```python
from build123d import *

# Parameters (mm, degrees)
SKETCH1_W          = 277
SKETCH1_H          = 97.5
BASE_FLANGE1_DEPTH = 1
JOG1_START         = -138.5
JOG1_DEPTH         = 277
JOG1_2_DEPTH       = 277
JOG2_START         = -138.5
JOG2_DEPTH         = 277
JOG2_2_DEPTH       = 277
SKETCH11_W         = 67
SKETCH11_H         = 15
SKETCH11_W_2       = 75
SKETCH11_W_3       = 77
CUT_EXTRUDE1_DEPTH = 148.204152455
SKETCH16_W         = 12
SKETCH16_H         = 22.35
TAB1_DEPTH         = 1
JOG4_START         = 126.5
JOG4_DEPTH         = 12
JOG4_2_DEPTH       = 12
SKETCH22_R         = 1.5
SCREW_HOLES_DEPTH  = 148.204152455
FILLET1_R          = 6
FILLET2_R          = 2


# Read off the part's stored shape, not the designer's step: Jog1, Jog2, Jog4
# Sheet-metal steps are written as plain solids
with BuildPart() as part:
    # Sketch1 → Base-Flange1 (new body)
    with BuildSketch(Plane.XY):
        Rectangle(SKETCH1_W, SKETCH1_H)
    extrude(amount=-BASE_FLANGE1_DEPTH)

    # Jog1 outline → Jog1 (cut)
    with BuildSketch(Plane.YZ.offset(JOG1_START)):
        with BuildLine():
            ThreePointArc((36.928097245, -1), (35.928097245, -0.732050807), (35.196046438, 0))
            Line((35.196046438, 0), (-48.75, 0))
            Line((-48.75, 0), (-48.75, -1))
            Line((-48.75, -1), (36.928097245, -1))
        make_face()
    extrude(amount=JOG1_DEPTH, mode=Mode.SUBTRACT)

    # Jog1 2 outline → Jog1 2 (add)
    with BuildSketch(Plane.YZ.offset(JOG1_START)):
        with BuildLine():
            Line((34.928097245, 7.5), (34.928097245, 1))
            ThreePointArc((34.928097245, 1), (34.996245593, 0.48236191), (35.196046438, 0))
            Line((35.196046438, 0), (36.928097245, 0))
            ThreePointArc((36.928097245, 0), (36.220990464, 0.292893219), (35.928097245, 1))
            Line((35.928097245, 1), (35.928097245, 7.5))
            ThreePointArc((35.928097245, 7.5), (35.342310807, 8.914213562), (33.928097245, 9.5))
            Line((33.928097245, 9.5), (-48.75, 9.5))
            Line((-48.75, 9.5), (-48.75, 8.5))
            Line((-48.75, 8.5), (33.928097245, 8.5))
            ThreePointArc((33.928097245, 8.5), (34.635204026, 8.207106781), (34.928097245, 7.5))
        make_face()
    extrude(amount=JOG1_2_DEPTH)

    # Jog2 outline → Jog2 (cut)
    with BuildSketch(Plane.YZ.offset(JOG2_START)):
        with BuildLine():
            Line((-48.75, 8.5), (-36.303953562, 8.5))
            ThreePointArc((-36.303953562, 8.5), (-35.571902755, 9.232050807), (-34.571902755, 9.5))
            Line((-34.571902755, 9.5), (-48.75, 9.5))
            Line((-48.75, 9.5), (-48.75, 8.5))
        make_face()
    extrude(amount=JOG2_DEPTH, mode=Mode.SUBTRACT)

    # Jog2 2 outline → Jog2 2 (add)
    with BuildSketch(Plane.YZ.offset(JOG2_START)):
        with BuildLine():
            Line((-48.75, -1), (-37.571902755, -1))
            ThreePointArc((-37.571902755, -1), (-36.157689193, -0.414213562), (-35.571902755, 1))
            Line((-35.571902755, 1), (-35.571902755, 7.5))
            ThreePointArc((-35.571902755, 7.5), (-35.279009536, 8.207106781), (-34.571902755, 8.5))
            Line((-34.571902755, 8.5), (-36.303953562, 8.5))
            ThreePointArc((-36.303953562, 8.5), (-36.503754407, 8.01763809), (-36.571902755, 7.5))
            Line((-36.571902755, 7.5), (-36.571902755, 1))
            ThreePointArc((-36.571902755, 1), (-36.864795974, 0.292893219), (-37.571902755, 0))
            Line((-37.571902755, 0), (-48.75, 0))
            Line((-48.75, 0), (-48.75, -1))
        make_face()
    extrude(amount=JOG2_2_DEPTH)

    # Sketch11 → Cut-Extrude1 (cut, through all)
    with BuildSketch(Plane(origin=(0, 0, -1), x_dir=(-1, 0, 0), z_dir=(0, 0, -1))):
        Polygon((-138.5, -48.75), (-123.5, -48.75), (-111.5, -48.75), (47.5, -48.75), (47.5, -33.75), (-111.5, -33.75), (-123.5, -33.75), (-123.5, -28.75), (-138.5, -28.75), align=None)
        with Locations((93, -41.25)):
            Rectangle(SKETCH11_W, SKETCH11_H)
        with Locations((-89, 41.25)):
            Rectangle(SKETCH11_W_2, SKETCH11_H)
        with Locations((-1, 41.25)):
            Rectangle(SKETCH11_W_3, SKETCH11_H)
        with Locations((88, 41.25)):
            Rectangle(SKETCH11_W_3, SKETCH11_H)
    extrude(amount=-CUT_EXTRUDE1_DEPTH, mode=Mode.SUBTRACT)

    # Sketch16 → Tab1 (add)
    with BuildSketch(Plane(origin=(0, 0, 8.5), x_dir=(-1, 0, 0), z_dir=(0, 0, -1))):
        with Locations((-132.5, -39.925)):
            Rectangle(SKETCH16_W, SKETCH16_H)
    extrude(amount=-TAB1_DEPTH)

    # Jog4 outline → Jog4 (cut)
    with BuildSketch(Plane.YZ.offset(JOG4_START)):
        with BuildLine():
            Line((-51.1, 8.5), (-30.986067978, 8.5))
            ThreePointArc((-30.986067978, 8.5), (-29.974744872, 9.238612788), (-28.75, 9.5))
            Line((-28.75, 9.5), (-51.1, 9.5))
            Line((-51.1, 9.5), (-51.1, 8.5))
        make_face()
    extrude(amount=JOG4_DEPTH, mode=Mode.SUBTRACT)

    # Jog4 2 outline → Jog4 2 (add)
    with BuildSketch(Plane.YZ.offset(JOG4_START)):
        with BuildLine():
            Line((-43.746018366, -1), (-33.75, -1))
            ThreePointArc((-33.75, -1), (-31.628679656, -0.121320344), (-30.75, 2))
            Line((-30.75, 2), (-30.75, 6.5))
            ThreePointArc((-30.75, 6.5), (-30.164213562, 7.914213562), (-28.75, 8.5))
            Line((-28.75, 8.5), (-30.986067978, 8.5))
            ThreePointArc((-30.986067978, 8.5), (-31.552517077, 7.570466269), (-31.75, 6.5))
            Line((-31.75, 6.5), (-31.75, 2))
            ThreePointArc((-31.75, 2), (-32.335786438, 0.585786438), (-33.75, 0))
            Line((-33.75, 0), (-43.746018366, 0))
            Line((-43.746018366, 0), (-43.746018366, -1))
        make_face()
    extrude(amount=JOG4_2_DEPTH)

    # Sketch22 → SCREW HOLES (cut, through all)
    with BuildSketch(Plane(origin=(0, 0, -1), x_dir=(-1, 0, 0), z_dir=(0, 0, -1))):
        with Locations((132.5, 42.75)):
            Circle(SKETCH22_R)
        with Locations((132.5, -42.75)):
            Circle(SKETCH22_R)
        with Locations((43.5, 42.75)):
            Circle(SKETCH22_R)
        with Locations((53.5, -42.75)):
            Circle(SKETCH22_R)
        with Locations((-45.5, 42.75)):
            Circle(SKETCH22_R)
        with Locations((-132.5, 42.75)):
            Circle(SKETCH22_R)
        with Locations((-132.5, -37.75)):
            Circle(SKETCH22_R)
    extrude(amount=-SCREW_HOLES_DEPTH, mode=Mode.SUBTRACT)

    # Fillet1
    fillet1_edges = [part.edges().sort_by_distance(p)[0] for p in [
        (39.5, 48.75, -0.5),
        (51.5, 48.75, -0.5),
        (-49.5, 48.75, -0.5),
        (-37.5, 48.75, -0.5),
        (-126.5, 48.75, -0.5),
        (-138.5, 48.75, -0.5),
        (-138.5, -48.75, -0.5),
        (-126.5, -48.75, -0.5),
        (-47.5, -48.75, -0.5),
        (-59.5, -48.75, -0.5),
        (138.5, -43.746018366, -0.5),
        (126.5, -43.746018366, -0.5),
        (138.5, 48.75, -0.5),
        (126.5, 48.75, -0.5),
    ]]
    fillet(fillet1_edges, radius=FILLET1_R - 0.0001)  # a hair under: the kernel refuses the full size

    # Fillet2
    fillet2_edges = [part.edges().sort_by_distance(p)[0] for p in [
        (123.5, -28.75, 9),
        (123.5, -33.75, 9),
    ]]
    fillet(fillet2_edges, radius=FILLET2_R)


solid = part.part
```
CAD build for the part. Positions are in the model's coordinates, mm. A direction names the side the tool comes from. Round coordinates to 2 decimals unless told otherwise and drop trailing zeros. Loops run counter-clockwise (first coordinate to the right, second up) from the corner with the lowest first, then second, coordinate; pieces in that order, holes last. Notation, with made-up numbers: M 70,-7.75 L 96,-7.75 A28 cw 96,19.25 Z; hole C 84.5,2 d11. An arc over 180 degrees is marked long. Use a Markdown table: item, result. Add a question column.
(1) Cut at A-A (x = 113.5). Give the cut face in (y, z).
(2) Cut at B-B (y = 9.5). Give the cut face in (x, z), and give its area (3 significant figures).
(3) Drill centre lines: line 1 (X direction, y = 35, z = 8.5); line 2 (Y direction, x = 45.5, z = -0.7); line 3 (Y direction, x = -132.5, z = -0.65). Where is each one in solid material? Low to high.
(4) Which spindle directions (+Z, -Z, +X, -X, +Y, -Y) get a long thin tool onto all of the face, cutting with end or side? Do faces 1 (the face through (-128.211, 46.946, -0.493)), 2 (the face through (-57.789, -46.946, -0.493)), 3 (the face through (-54, -36.572, 4)), 4 (the face through (-133, 35.928, 4)). Say none if no direction does.
(5) Flat gauge pins, fed straight in: pin 1 (5 mm diameter, centred on x = -54.5, y = -24, fed in from -Z); pin 2 (0.8 mm diameter, centred on x = -0.5, z = 9, fed in from +Y); pin 3 (9.5 mm diameter, centred on x = -135.5, y = 41, fed in from +Z) (3 decimals). Where does each tip first touch, or does it go through?
(6) Pull direction Y, two halves, no side cores. Call faces 5 (the face through (136.696, -42.035, -0.507)), 6 (the face through (-133, 34.928, 4)), 7 (the face through (-136.789, 46.946, -0.507)): +Y half, -Y half, draft (parallel to the pull), parting line (faces both ways), or undercut.
Geometry says:
| question | item | result |
|---|---|---|
| 1 | outline | M -33.75,8.5 L 33.75,8.5 L 33.75,9.5 L -33.75,9.5 Z |
| 2 | outline | M -138.5,8.5 L 138.5,8.5 L 138.5,9.5 L -138.5,9.5 Z |
| 2 | area | 277 mm² |
| 3 | line 1 | x = -138.5 to -126.5, -49.5 to -37.5, 39.5 to 51.5, 126.5 to 138.5 |
| 3 | line 2 | y = 35.87 to 41.25, 44.25 to 48.75 |
| 3 | line 3 | y = -48.75 to -44.25, -41.25 to -36.44, 35.8 to 41.25, 44.25 to 48.75 |
| 4 | face 1 | +Z, -Z, +Y |
| 4 | face 2 | +Z, -Z, -Y |
| 4 | face 3 | +Z, +X, -X, -Y |
| 4 | face 4 | +Z, +X, -X, +Y |
| 5 | pin 1 | stops at z = 8.5 |
| 5 | pin 2 | stops at y = 33.75 |
| 5 | pin 3 | stops at z = 0.265 |
| 6 | face 5 | -Y half |
| 6 | face 6 | undercut |
| 6 | face 7 | +Y half |
